Here's how the part is built. I have some questions about the finished solid (model axes, mm). A direction names the side the tool comes from. Give positions to 0.01 mm unless a question says otherwise; leave off trailing zeros. Loops run counter-clockwise (first coordinate to the right, second up) from the corner with the lowest first, then second, coordinate; pieces in that order, holes last.
Q1. Will these pins go through, and if not, where does the flat tip stop? P1, Ø8, axis at y = -14, z = 28, coming from the +X side; P2, Ø10, axis at y = -40.5, z = 24.5, coming from the +X side; P3, Ø1.5, axis at y = -17.5, z = 1.5, coming from the +X side.
Q2. We'd pull the mould along Z, two halves only. Please class faces 1 (the face through (8.497, -25, 36)), 2 (the face through (45.926, -25.044, 10.947)), 3 (the face through (9.627, -25.044, 29.494)), 4 (the face through (16, -25, 20.91)): +Z half, -Z half, draft (parallel to the pull), parting line (faces both ways), or undercut.
Q3. For faces 5 (the face through (17, -25, -4.296)), 6 (the face through (27, 0, 9)), 7 (the face through (14.99, -25, -19)), 8 (the face through (27, -50.8, 9)), 9 (the face through (15, -25, 29.693)), which set-ups out of +Z, -Z, +X, -X, +Y, -Y let a thin tool reach every point of the face, with its end or its side?
Q4. I need wall thicknesses on line 1 (Z direction, x = 18, y = -6); line 2 (Z direction, x = 17.5, y = -4); line 3 (X direction, y = -18, z = 8). Which ranges of each line are inside material? Lowest first, please.
Q5. If we section it at B-B (x = 36): Please give me the cut outline in (y, z).
Q6. If we section it at C-C (z = -3): Please give me the cut outline in (x, y).
Q7. If we section it at A-A (y = -24): Please give me the cut outline in (x, z).
from build123d import *

# Parameters (mm, degrees)
F1_DEPTH = 50.8


with BuildPart() as f1:
    # F0 (on Front) → F1 (new body)
    with BuildSketch(Plane.XZ):
        with BuildLine():
            Line((14.989941, -12.698484), (14.989941, -26.06531))
            ThreePointArc((14.989941, -26.06531), (45.86306, 11.702062), (8.497481, 43.060273))
            Line((8.497481, 43.060273), (10.788937, 29.693447))
            Line((10.788937, 29.693447), (18.427124, 29.693447))
            Line((18.427124, 29.693447), (18.427124, 20.909535))
            Line((18.427124, 20.909535), (12.889439, 20.909535))
            Line((12.889439, 20.909535), (12.889439, -4.29648))
            Line((12.889439, -4.29648), (20.71858, -4.29648))
            Line((20.71858, -4.29648), (20.71858, -12.698484))
            Line((20.71858, -12.698484), (14.989941, -12.698484))
        make_face()
        Polygon((10.788937, 29.693447), (8.497481, 43.060273), (8.497481, 29.300626), align=None)
    extrude(amount=F1_DEPTH)


solid = f1.part
Check sheet entries:
1. P1: stops at x = 42.34
1. P2: stops at x = 44.21
1. P3: stops at x = 45.46
2. face 1: draft
2. face 2: parting line
2. face 3: -Z half
2. face 4: undercut
3. face 5: -X, +Y, -Y
3. face 6: +Z, -Z, +X, -X, +Y
3. face 7: -Z, -X, +Y, -Y
3. face 8: +Z, -Z, +X, -X, -Y
3. face 9: +Y, -Y
4. line 1: z = -25.61 to -12.7, -4.3 to 20.91, 29.69 to 42.52
4. line 2: z = -25.7 to -12.7, -4.3 to 20.91, 29.69 to 42.61
4. line 3: x = 12.89 to 46.01
5. outline: (-50.8, -15.94) - (0, -15.94) - (0, 32.85) - (-50.8, 32.85) - close
6. outline: (12.89, -50.8) - (44.07, -50.8) - (44.07, 0) - (12.89, 0) - close
7. outline: (8.5, 29.3) - (10.79, 29.69) - (18.43, 29.69) - (18.43, 20.91) - (12.89, 20.91) - (12.89, -4.3) - (20.72, -4.3) - (20.72, -12.7) - (14.99, -12.7) - (14.99, -26.07) arc R34.72 ccw to (8.5, 43.06) - close
